The model under review builds one solid part; all positions refer to its coordinate system, in mm. A direction names the side the tool comes from. Give positions to 0.01 mm unless a question says otherwise; leave off trailing zeros. Order: outer loops, then holes, each group sorted by start corner. A loop starts at its lowest first (then second) coordinate and runs counter-clockwise, first axis right, second up.
```python
from build123d import *

# Parameters (mm, degrees)
F0_W          = 300
F0_H          = 210
F1_DEPTH      = 157.14
F1_DEPTH_BACK = 157.14
F3_DEPTH      = 105
F3_DEPTH_BACK = 105
F4_R          = 4.5
F5_DEPTH      = 21
F6_R          = 6.5
F6_R_2        = 4.25
F7_DEPTH      = 20
F6_R_3        = 3
F8_DEPTH      = 10
F6_R_4        = 5
F9_DEPTH      = 40
F6_R_5        = 4
F10_DEPTH     = 16
F11_SIZE      = 25
F12_R         = 1.5875
F12_R_2       = 1.5
F13_DEPTH     = 10
F14_DEPTH     = 40
F15_R         = 1.5
F16_DEPTH     = 70
F17_R         = 1.5
F18_DEPTH     = 70
F20_DEPTH     = 2.7
F22_DEPTH     = 2.7
F23_R         = 4.5
F24_DEPTH     = 21


# Not quite as in the source:
# - a feature names something its author has since deleted; it is built from what else it names


with BuildPart() as f1:
    # F0 (on Top) → F1 (new body, two sides)
    with BuildSketch(Plane.XY) as f1_sk:
        Rectangle(F0_W, F0_H)
        with BuildLine():
            ThreePointArc((-50, -86), (-136, 0), (-50, 86))
            Line((-50, 86), (50, 86))
            ThreePointArc((50, 86), (136, 0), (50, -86))
            Line((50, -86), (-50, -86))
        make_face(mode=Mode.SUBTRACT)
        with BuildLine():
            Line((50, 86), (-50, 86))
            ThreePointArc((-50, 86), (-136, 0), (-50, -86))
            Line((-50, -86), (50, -86))
            ThreePointArc((50, -86), (136, 0), (50, 86))
        make_face()
        with BuildLine():
            ThreePointArc((-50, -81), (-131, 0), (-50, 81))
            Line((-50, 81), (50, 81))
            ThreePointArc((50, 81), (131, 0), (50, -81))
            Line((50, -81), (-50, -81))
        make_face(mode=Mode.SUBTRACT)
        with BuildLine():
            Line((50, 81), (-50, 81))
            ThreePointArc((-50, 81), (-131, 0), (-50, -81))
            Line((-50, -81), (50, -81))
            ThreePointArc((50, -81), (131, 0), (50, 81))
        make_face()
        with BuildLine():
            ThreePointArc((0, -54.6611964743), (-124.08, 0), (0, 54.6611964743))
            ThreePointArc((0, 54.6611964743), (124.08, 0), (0, -54.6611964743))
        make_face(mode=Mode.SUBTRACT)
    extrude(amount=F1_DEPTH)
    extrude(f1_sk.sketch, amount=-F1_DEPTH_BACK)

    # F2 (on Front) → F3 (cut, two sides)
    with BuildSketch(Plane.XZ) as f3_sk:
        with BuildLine():
            ThreePointArc((12.5, 119.64), (0, 132.14), (-12.5, 119.64))
            Line((-12.5, 119.64), (-12.5, -119.64))
            ThreePointArc((-12.5, -119.64), (0, -132.14), (12.5, -119.64))
            Line((12.5, -119.64), (12.5, 119.64))
        make_face()
    extrude(amount=-F3_DEPTH, mode=Mode.SUBTRACT)
    extrude(f3_sk.sketch, amount=F3_DEPTH_BACK, mode=Mode.SUBTRACT)

    # F4 (on face) → F5 (cut)
    with BuildSketch(Plane.XZ.offset(105)):
        with Locations((-31.4, 112)):
            Circle(F4_R)
        with Locations((-31.4, 56)):
            Circle(F4_R)
        with Locations((-31.4, 0)):
            Circle(F4_R)
        with Locations((-31.4, -56)):
            Circle(F4_R)
        with Locations((-31.4, -112)):
            Circle(F4_R)
        with Locations((31.4, -112)):
            Circle(F4_R)
        with Locations((31.4, -56)):
            Circle(F4_R)
        with Locations((31.4, 0)):
            Circle(F4_R)
        with Locations((31.4, 56)):
            Circle(F4_R)
        with Locations((31.4, 112)):
            Circle(F4_R)
    extrude(amount=-F5_DEPTH, mode=Mode.SUBTRACT)

    # F6 (on face) → F7 (cut)
    with BuildSketch(Plane.XY.offset(157.14)):
        with Locations((140, 50)):
            Circle(F6_R)
        with Locations((140, 50)):
            Circle(F6_R_2, mode=Mode.SUBTRACT)
        with Locations((140, -50)):
            Circle(F6_R)
        with Locations((140, -50)):
            Circle(F6_R_2, mode=Mode.SUBTRACT)
        with Locations((70, -95)):
            Circle(F6_R)
        with Locations((70, -95)):
            Circle(F6_R_2, mode=Mode.SUBTRACT)
        with Locations((-70, -95)):
            Circle(F6_R)
        with Locations((-70, -95)):
            Circle(F6_R_2, mode=Mode.SUBTRACT)
        with Locations((-140, -50)):
            Circle(F6_R)
        with Locations((-140, -50)):
            Circle(F6_R_2, mode=Mode.SUBTRACT)
        with Locations((-140, 50)):
            Circle(F6_R)
        with Locations((-140, 50)):
            Circle(F6_R_2, mode=Mode.SUBTRACT)
        with Locations((-70, 95)):
            Circle(F6_R)
        with Locations((-70, 95)):
            Circle(F6_R_2, mode=Mode.SUBTRACT)
        with Locations((70, 95)):
            Circle(F6_R)
        with Locations((70, 95)):
            Circle(F6_R_2, mode=Mode.SUBTRACT)
    extrude(amount=-F7_DEPTH, mode=Mode.SUBTRACT)

    # F6 (on face) → F8 (cut)
    with BuildSketch(Plane.XY.offset(157.14)):
        with Locations((-50, 95)):
            Circle(F6_R_3)
        with Locations((-145, 0)):
            Circle(F6_R_3)
        with Locations((50, 95)):
            Circle(F6_R_3)
        with Locations((145, 0)):
            Circle(F6_R_3)
        with Locations((-50, -95)):
            Circle(F6_R_3)
        with Locations((50, -95)):
            Circle(F6_R_3)
    extrude(amount=-F8_DEPTH, mode=Mode.SUBTRACT)

    # F6 (on face) → F9 (cut)
    with BuildSketch(Plane.XY.offset(157.14)):
        with Locations((-70, 95)):
            Circle(F6_R_2)
        with Locations((-140, 50)):
            Circle(F6_R_2)
        with Locations((-140, -50)):
            Circle(F6_R_2)
        with Locations((-70, -95)):
            Circle(F6_R_2)
        with Locations((70, -95)):
            Circle(F6_R_2)
        with Locations((140, -50)):
            Circle(F6_R_2)
        with Locations((140, 50)):
            Circle(F6_R_2)
        with Locations((70, 95)):
            Circle(F6_R_2)
        with Locations((-140, 70)):
            Circle(F6_R_4)
        with Locations((140, -70)):
            Circle(F6_R_4)
    extrude(amount=-F9_DEPTH, mode=Mode.SUBTRACT)

    # F6 (on face) → F10 (cut)
    with BuildSketch(Plane.XY.offset(157.14)):
        with Locations((-120, 90)):
            Circle(F6_R_5)
        with Locations((-120, -90)):
            Circle(F6_R_5)
        with Locations((120, -90)):
            Circle(F6_R_5)
        with Locations((120, 90)):
            Circle(F6_R_5)
    extrude(amount=-F10_DEPTH, mode=Mode.SUBTRACT)

    # F11
    f11_edges = [f1.edges().sort_by_distance(p)[0] for p in [
        (-150, 105, 0),
        (-150, -105, 0),
        (150, 105, 0),
        (150, -105, 0),
    ]]
    chamfer(f11_edges, length=F11_SIZE)

    # F12 (on face) → F13 (cut)
    with BuildSketch(Plane.YZ.offset(150)):
        Circle(F12_R)
        Circle(F12_R_2, mode=Mode.SUBTRACT)
    extrude(amount=-F13_DEPTH, mode=Mode.SUBTRACT)

    # F14 (cut): a face of the model
    f14_faces = [f1.faces().sort_by_distance(p)[0] for p in [
        (150, 0, 0),
    ]]
    extrude(f14_faces, amount=-F14_DEPTH, mode=Mode.SUBTRACT)

    # F15 (on face) → F16 (cut)
    with BuildSketch(Plane(origin=(115, -115, 0), x_dir=(0.7071067812, 0.7071067812, 0), z_dir=(0.7071067812, -0.7071067812, 0))):
        with Locations((31.8221356237, 0)):
            Circle(F15_R)
    extrude(amount=-F16_DEPTH, mode=Mode.SUBTRACT)

    # F17 (on face) → F18 (cut)
    with BuildSketch(Plane(origin=(115, 115, 0), x_dir=(-0.7071067812, 0.7071067812, 0), z_dir=(0.7071067812, 0.7071067812, 0))):
        with Locations((-31.8174746831, 0)):
            Circle(F17_R)
    extrude(amount=-F18_DEPTH, mode=Mode.SUBTRACT)

    # F19 (on face) → F20 (cut)
    with BuildSketch(Plane.XY.offset(157.14)):
        with BuildLine():
            Line((-50, -86), (50, -86))
            ThreePointArc((50, -86), (136, 0), (50, 86))
            Line((50, 86), (-50, 86))
            ThreePointArc((-50, 86), (-136, 0), (-50, -86))
        make_face()
        with BuildLine():
            ThreePointArc((50, 81), (131, 0), (50, -81))
            Line((50, -81), (-50, -81))
            ThreePointArc((-50, -81), (-131, 0), (-50, 81))
            Line((-50, 81), (50, 81))
        make_face(mode=Mode.SUBTRACT)
    extrude(amount=-F20_DEPTH, mode=Mode.SUBTRACT)

    # F21 (on face) → F22 (cut)
    with BuildSketch(Plane(origin=(0, 0, -157.14), x_dir=(1, 0, 0), z_dir=(0, 0, -1))):
        with BuildLine():
            Line((50, 86), (-50, 86))
            ThreePointArc((-50, 86), (-136, 0), (-50, -86))
            Line((-50, -86), (50, -86))
            ThreePointArc((50, -86), (136, 0), (50, 86))
        make_face()
        with BuildLine():
            ThreePointArc((-50, -81), (-131, 0), (-50, 81))
            Line((-50, 81), (50, 81))
            ThreePointArc((50, 81), (131, 0), (50, -81))
            Line((50, -81), (-50, -81))
        make_face(mode=Mode.SUBTRACT)
    extrude(amount=-F22_DEPTH, mode=Mode.SUBTRACT)

    # F23 (on face) → F24 (cut)
    with BuildSketch(Plane(origin=(0, 105, 0), x_dir=(-1, 0, 0), z_dir=(0, 1, 0))):
        with Locations((32.3209376876, -110.7883939175)):
            Circle(F23_R)
        with Locations((-30.4790623124, -110.7883939175)):
            Circle(F23_R)
        with Locations((32.3209376876, -54.7883939175)):
            Circle(F23_R)
        with Locations((32.3209376876, 1.2116060825)):
            Circle(F23_R)
        with Locations((32.3209376876, 57.2116060825)):
            Circle(F23_R)
        with Locations((32.3209376876, 113.2116060825)):
            Circle(F23_R)
        with Locations((-30.4790623124, 113.2116060825)):
            Circle(F23_R)
        with Locations((-30.4790623124, 57.2116060825)):
            Circle(F23_R)
        with Locations((-30.4790623124, 1.2116060825)):
            Circle(F23_R)
        with Locations((-30.4790623124, -54.7883939175)):
            Circle(F23_R)
    extrude(amount=-F24_DEPTH, mode=Mode.SUBTRACT)


solid = f1.part
```
1. For faces 4 (the cylindrical face through (26.2, 94.6, -53.4)), 5 (the cylindrical face through (-31.99, -94.65, 116.46)), 6 (the flat face through (-70, 95, 117.14)), 7 (the cylindrical face through (130.98, -1.78, -155.81)), list the 3-axis set-ups (+Z, -Z, +X, -X, +Y, -Y) from which the entire face can be reached by the end or side of a thin tool; tool diameter is ignored.
2. Insertion check: pin 1 (6 mm diameter, centred on x = -140, y = 70, fed in from +Z); pin 2 (7 mm diameter, centred on x = 69.5, y = 96.5, fed in from +Z); pin 3 (2.5 mm diameter, centred on x = 119, y = 90, fed in from +Z). Each pin has a flat end and moves straight along its axis. Give the tip position at first contact, or say it passes through.
3. Take a section at D-D (x = 120). Count the separate pieces of the cut face and the enclosed holes in it, and give its area (3 significant figures).
4. Take a section at B-B (y = 38). Write out the cut boundary in (x, z).
5. Take a section at A-A (z = 74). Write out the cut boundary in (x, y), and give its area (3 significant figures).
6. Draft analysis for pull direction Y (two halves, no side actions). For faces 1 (the cylindrical face through (-34.72, -94.65, 3.04)), 2 (the cylindrical face through (-135.98, 1.89, 155.81)), 3 (the flat face through (31, -84, 112)), state which applies: pulls with the +Y half, pulls with the -Y half, needs draft (parallel to the pull), parting line crosses it, or undercut.
7. To check wall thickness, follow line 1 (Y direction, x = -50, z = 154); line 2 (Z direction, x = -31.4, y = -96); line 3 (X direction, y = 2, z = 9.5). State the ranges of each line that lie inside material, in increasing order.
8. Take a section at C-C (x = 59.5). Write out the cut boundary in (y, z).
Answer:
1. face 4: +Y
1. face 5: -Y
1. face 6: +Z
1. face 7: -Z
2. pin 1: stops at z = 117.14
2. pin 2: stops at z = 137.14
2. pin 3: stops at z = 141.14
3. separate pieces: 2
3. enclosed holes: 2
3. area: 50,400 mm2
4. outline: (-150, -157.14) - (-127.15, -157.14) - (-127.15, -154.44) - (-121.53, -154.44) - (-121.53, -157.14) - (-113.59, -157.14) - (-113.59, 157.14) - (-121.53, 157.14) - (-121.53, 154.44) - (-127.15, 154.44) - (-127.15, 157.14) - (-150, 157.14) - close; (113.59, -157.14) - (121.53, -157.14) - (121.53, -154.44) - (127.15, -154.44) - (127.15, -157.14) - (150, -157.14) - (150, 157.14) - (127.15, 157.14) - (127.15, 154.44) - (121.53, 154.44) - (121.53, 157.14) - (113.59, 157.14) - close
5. outline: (-150, -80) - (-125, -105) - (-12.5, -105) - (-12.5, -63.89) arc R74.08 cw (long way) to (-12.5, 63.89) - (-12.5, 105) - (-125, 105) - (-150, 80) - close; (12.5, -105) - (125, -105) - (150, -80) - (150, 80) - (125, 105) - (12.5, 105) - (12.5, 63.89) arc R74.08 cw (long way) to (12.5, -63.89) - close
5. area: 28,600 mm2
6. face 1: needs draft
6. face 2: undercut
6. face 3: pulls with the -Y half
7. line 1: y = -105 to -98, -92 to -74.08, 74.08 to 92, 98 to 105
7. line 2: z = -157.14 to -116.5, -107.5 to -60.5, -51.5 to -4.5, 4.5 to 51.5, 60.5 to 107.5, 116.5 to 157.14
7. line 3: x = -150 to -124.05, 124.05 to 150
8. outline: (-105, -157.14) - (-85.47, -157.14) - (-85.47, -154.44) - (-80.44, -154.44) - (-80.44, -157.14) - (-73.47, -157.14) - (-73.47, 157.14) - (-80.44, 157.14) - (-80.44, 154.44) - (-85.47, 154.44) - (-85.47, 157.14) - (-105, 157.14) - close; (73.47, -157.14) - (80.44, -157.14) - (80.44, -154.44) - (85.47, -154.44) - (85.47, -157.14) - (105, -157.14) - (105, 157.14) - (85.47, 157.14) - (85.47, 154.44) - (80.44, 154.44) - (80.44, 157.14) - (73.47, 157.14) - close
